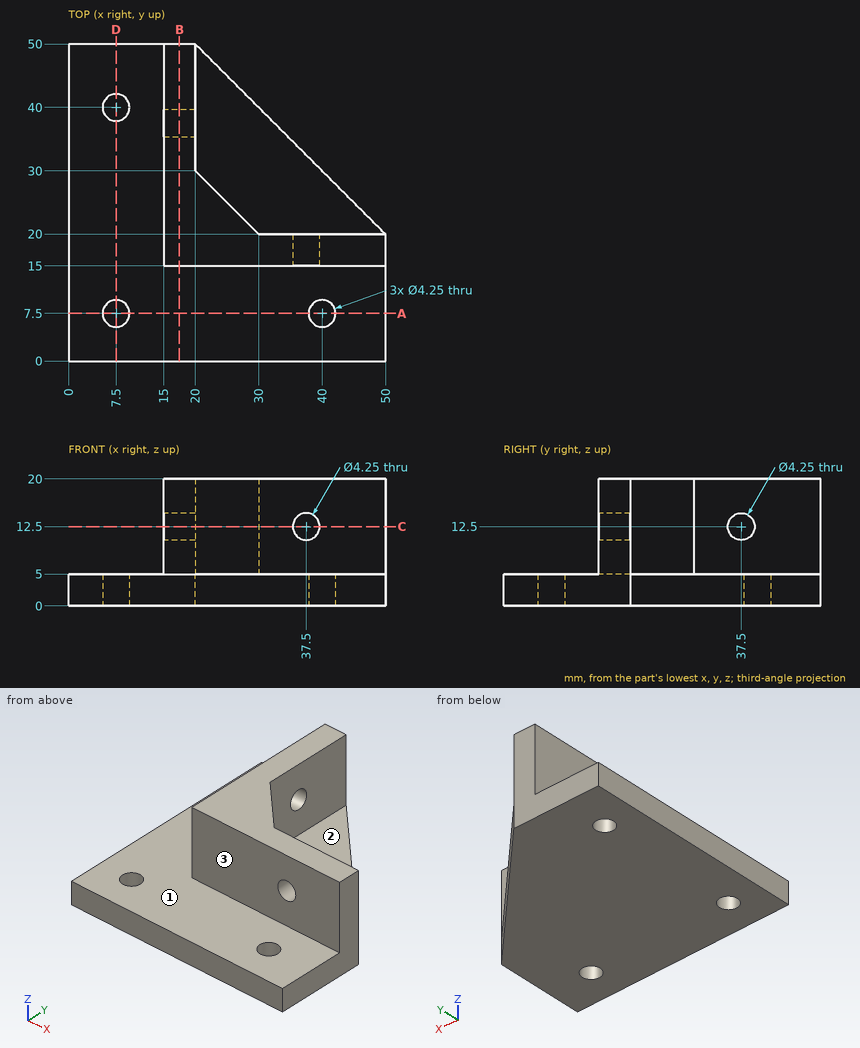
Input: dimensioned drawing with shaded views. Units: mm. Origin: part minimum x, y, z. A direction names the side the tool comes from. Coordinates: 2 decimals unless noted, no trailing zeros. Order: outer loops, then holes, each group sorted by start corner. A loop starts at its lowest first (then second) coordinate and runs counter-clockwise, first axis right, second up. Notation, with made-up numbers: M 75,79 L 131,79 A25 cw 131,114 Z; hole C -13,-14 d4. An arc over 180 degrees is marked long. Answer as CSV lines item,"result".
Q1. Set-up query: the marked faces 1, 2 and 3. Return all of +Z, -Z, +X, -X, +Y, -Y with unobstructed straight access to the full face (end or side cutting, diameter ignored); none if empty.
Answers:
face 1,"+Z, -X, -Y"
face 2,"+Z, +X, +Y"
face 3,"+Z, +X, -X, -Y"
Q2. First-contact query: P1, Ø7.5, axis at x = 40, z = 15.5, coming from the -Y side; P2, Ø4.5, axis at x = 41.5, z = 14, coming from the +Y side; P3, Ø5, axis at x = 40, y = 7.5, coming from the +Z side. Flat tips, straight axial feed; report the tip coordinate or a pass-through.
Answers:
P1,"stops at y = 15"
P2,"stops at y = 20"
P3,"stops at z = 5"
Q3. Line query: probe 1 along Y at (x, z) = (7.5, 3.2) (3 decimals); probe 2 along Z at (x, y) = (12, 17.5); probe 3 along Y at (x, z) = (47.5, 5.25). Output: solid intervals per line, ascending. Write a range as [from, to].
Answers:
probe 1,"y = [0, 5.375], [9.625, 37.875], [42.125, 50]"
probe 2,"z = [0, 5]"
probe 3,"y = [15, 20]"
Q4. Section A-A on y = 7.5. Return the cut outline in (x, z) (3 decimals), and give its area (4 significant figures).
Answers:
outline,"M 0,0 L 5.375,0 L 5.375,5 L 0,5 Z; M 9.625,0 L 37.875,0 L 37.875,5 L 9.625,5 Z; M 42.125,0 L 50,0 L 50,5 L 42.125,5 Z"
area,"207.5 mm^2"
Q5. Section B-B on x = 17.5. Return the cut outline in (y, z) (3 decimals), and give its area (3 significant figures).
Answers:
outline,"M 0,0 L 50,0 L 50,20 L 15,20 L 15,5 L 0,5 Z; hole C 37.5,12.5 d4.25"
area,"761 mm^2"
Q6. Section C-C on z = 12.5. Return the cut outline in (x, y) (3 decimals).
Answers:
outline,"M 15,15 L 35.375,15 L 35.375,20 L 30,20 L 20,30 L 20,35.375 L 15,35.375 Z; M 15,39.625 L 20,39.625 L 20,50 L 15,50 Z; M 39.625,15 L 50,15 L 50,20 L 39.625,20 Z"
